Job drawing, mm, ordinate dimensions from the low corner. One solid piece. Give positions to 0.01 mm unless a question says otherwise; leave off trailing zeros. Write each loop counter-clockwise with the first axis right and the second up, starting at its lowest first coordinate (ties: lowest second). Pieces come first, ordered by that corner, then holes. Notation, with made-up numbers: (80, 36.25) - (96, 36.25) arc R10 ccw to (96, 46.25) - close; hole circle Ø9 at (27.25, 7.5). An arc over 180 degrees is marked (long way). Answer in a Markdown table with one row per item. Add a question column.
1. Drop a flat-ended pin along its axis: pin 1 Ø3 at (x, z) = (50, 45) entering from -Y. Give the stop position or say it passes through.
2. Band-saw the part on C-C on y = 5.75. State how many separate pieces and enclosed holes the cut face has, plus the area to 3 significant figures.
3. Probe line 1 along Z through (x, y) = (40, 2.5); line 2 along Z through (x, y) = (10, 4); line 3 along X through (y, z) = (3.5, 3). List the from-to ranges inside material, lowest first.
4. Band-saw the part on A-A on x = 10. Write the cut outline in (y, z).
5. Band-saw the part on B-B on z = 44. Write the cut outline in (x, y).
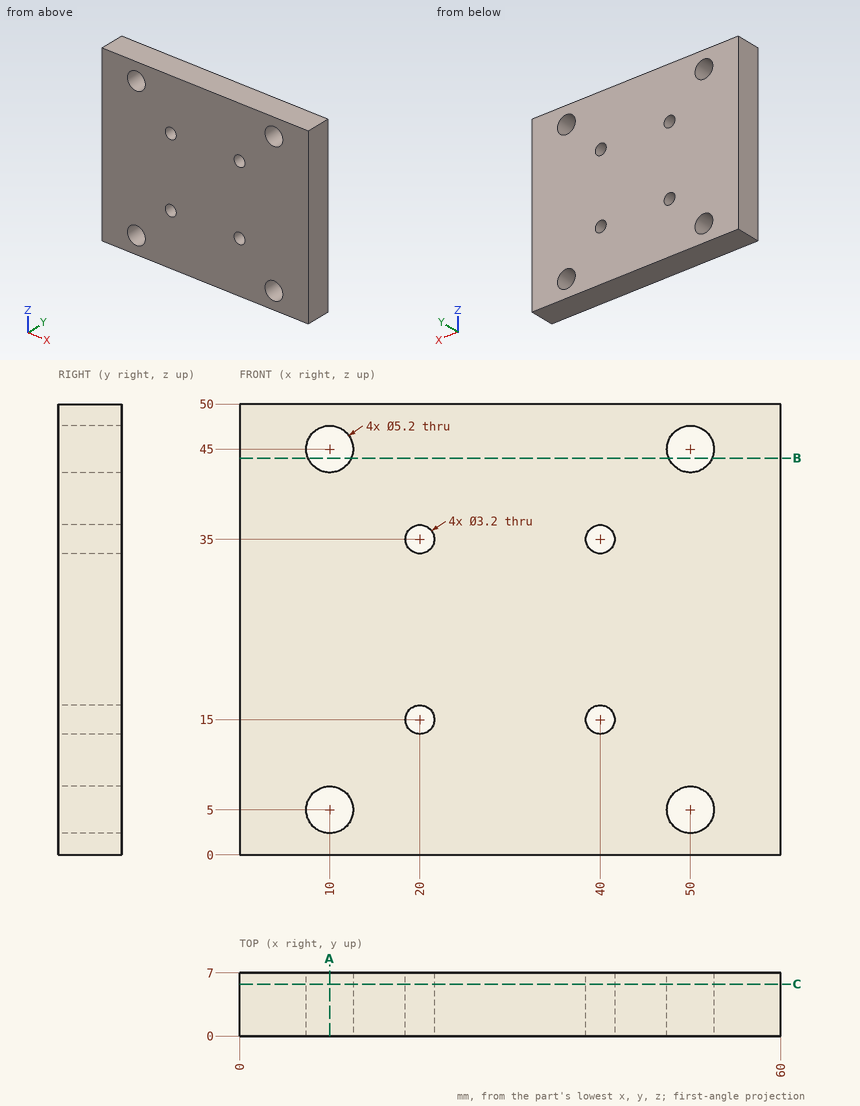
Values:
| question | item | result |
|---|---|---|
| 1 | pin 1 | passes through |
| 2 | separate pieces | 1 |
| 2 | enclosed holes | 8 |
| 2 | area | 2,880 mm² |
| 3 | line 1 | z = 0 to 13.4, 16.6 to 33.4, 36.6 to 50 |
| 3 | line 2 | z = 0 to 2.4, 7.6 to 42.4, 47.6 to 50 |
| 3 | line 3 | x = 0 to 8.34, 11.66 to 48.34, 51.66 to 60 |
| 4 | outline | (0, 0) - (7, 0) - (7, 2.4) - (0, 2.4) - close; (0, 7.6) - (7, 7.6) - (7, 42.4) - (0, 42.4) - close; (0, 47.6) - (7, 47.6) - (7, 50) - (0, 50) - close |
| 5 | outline | (0, 0) - (7.6, 0) - (7.6, 7) - (0, 7) - close; (12.4, 0) - (47.6, 0) - (47.6, 7) - (12.4, 7) - close; (52.4, 0) - (60, 0) - (60, 7) - (52.4, 7) - close |
